Verification items for the finished model (mm, model axes). A direction names the side the tool comes from. Coordinates: 2 decimals unless noted, no trailing zeros. Order: outer loops, then holes, each group sorted by start corner. A loop starts at its lowest first (then second) coordinate and runs counter-clockwise, first axis right, second up. Notation, with made-up numbers: M 77.5,-9 L 94.5,-9 A17 ccw 94.5,15 Z; hole C 54.5,64 d1. An arc over 180 degrees is marked long. Write item = value, one per line.
```python
from build123d import *

# Parameters (mm, degrees)
F0_W     = 1025
F0_H     = 400
F1_DEPTH = 400
F2_T     = -1
F5_D     = 40
F8_D     = 30


# Not quite as in the source:
# - the program builds the solid bodies; features that only make, move or delete a surface that nothing else refers to are left out


with BuildPart() as f1:
    # F0 (on Top) → F1 (new body)
    with BuildSketch(Plane.XY):
        Rectangle(F0_W, F0_H)
    extrude(amount=F1_DEPTH)

    # F2
    f2_openings = [f1.faces().sort_by_distance(p)[0] for p in [
        (0, 0, 400),
    ]]
    offset(amount=F2_T, openings=f2_openings)

    # F5 (through all)
    with Locations(Plane.XY.offset(1)):
        with Locations((489.5, 177), (489.5, -177), (-489.5, 177), (-489.5, -177)):
            Hole(F5_D / 2)

    # F8 (through all)
    with Locations(Plane(origin=(-512.5, 0, 0), x_dir=(0, -1, 0), z_dir=(-1, 0, 0))):
        with Locations((0, 50)):
            Hole(F8_D / 2)


solid = f1.part
```
Item 1: Tool access check on faces 1 (the cylindrical face through (512.007, -1.953, 64.872)), 2 (the flat face through (-511.5, -3, 198)). Record the directions out of +Z, -Z, +X, -X, +Y, -Y that give a thin tool (end or side, any length) a straight path to the whole face; none if there is none.
Report:
face_1 = +X, -X
face_2 = +Z
Item 2: Sectioned sample at B-B, the plane y = 177. Enter the section's corners in (x, z).
Report:
outline = M -512.5,0 L -509.5,0 L -509.5,1 L -511.5,1 L -511.5,400 L -512.5,400 Z; M -469.5,0 L 469.5,0 L 469.5,1 L -469.5,1 Z; M 509.5,0 L 512.5,0 L 512.5,400 L 511.5,400 L 511.5,1 L 509.5,1 Z
Item 3: Sectioned sample at A-A, the plane z = 50. Enter the section's corners in (x, y), then the cut area to 3 significant figures.
Report:
outline = M -512.5,-200 L 512.5,-200 L 512.5,-15 L 511.5,-15 L 511.5,-199 L -511.5,-199 L -511.5,-15 L -512.5,-15 Z; M -512.5,15 L -511.5,15 L -511.5,199 L 511.5,199 L 511.5,15 L 512.5,15 L 512.5,200 L -512.5,200 Z
area = 2,790 mm^2
Item 4: Scan lines: L1, parallel to X at y = -120, z = 152; L2, parallel to Y at x = -197, z = 319.5; L3, parallel to Y at x = 489.5, z = 0.45. Record each from-to range of solid material in increasing order. Write a range as from..to.
Report:
L1 = -512.5..-511.5, 511.5..512.5
L2 = -200..-199, 199..200
L3 = -200..-197, -157..157, 197..200
Item 5: Release check for a two-part mould opening along Z. For faces 3 (the cylindrical face through (-511.993, -1.953, 64.872)), 4 (the cylindrical face through (-500.252, 193.864, 0.493)), 5 (the flat face through (-7, 3, 0)) record: pulls with the +Z half, pulls with the -Z half, needs draft (parallel to the pull), parting line crosses it, or undercut.
Report:
face_3 = undercut
face_4 = needs draft
face_5 = pulls with the -Z half
Item 6: Gauge pin test, flat ends, axial feed: pin 1 (8 mm diameter, centred on x = -405, y = -2, fed in from -Z); pin 2 (3 mm diameter, centred on x = 186.5, y = 12, fed in from +Z). Record the tip position at first contact, or that the pin passes through.
Report:
pin_1 = 0
pin_2 = 1
Item 7: Sectioned sample at C-C, the plane x = -489.5. Enter the section's corners in (y, z).
Report:
outline = M -200,0 L -197,0 L -197,1 L -199,1 L -199,400 L -200,400 Z; M -157,0 L 157,0 L 157,1 L -157,1 Z; M 197,0 L 200,0 L 200,400 L 199,400 L 199,1 L 197,1 Z
Item 8: Sectioned sample at D-D, the plane y = 51. Enter the section's corners in (x, z).
Report:
outline = M -512.5,0 L 512.5,0 L 512.5,400 L 511.5,400 L 511.5,1 L -511.5,1 L -511.5,400 L -512.5,400 Z
